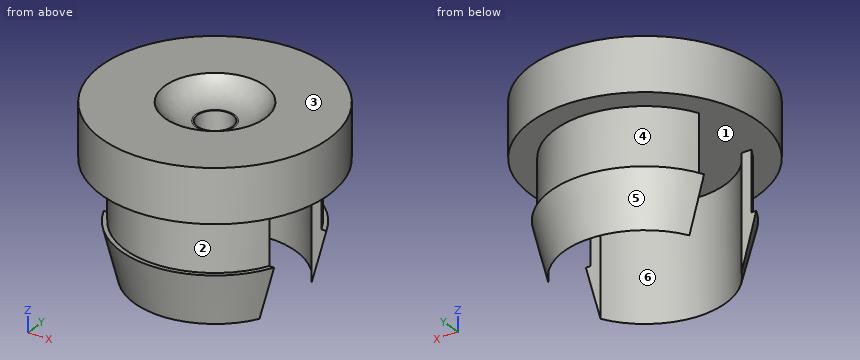
Autodesk Inventor part; units mm, degrees
ref_plane "XZ Plane" through (0, 0, 0) normal (0, 1, 0) x (-1, 0, 0)
ref_plane "XY Plane" through (0, 0, 0) normal (0, 0, 1) x (1, 0, 0)
sketch "Sketch1" plane through (0, 0, 0) normal (0, 0, 1) x (1, 0, 0)
  circle A0 centre (0, 0) radius 6.4
  dimension "d0" = 12.8
sketch "Sketch2" plane through (0, 0, 0) normal (0, 0, 1) x (1, 0, 0)
  circle A0 centre (0, 0) radius 2.825
  dimension "d3" = 5.65
sketch "Sketch3" plane through (0, 0, 0) normal (0, 0, 1) x (1, 0, 0)
  circle A0 centre (0, 0) radius 1
  dimension "d4" = 2
extrude "Extrusion1" add sketch "Sketch1" against normal blind 3
extrude "Extrusion2" cut sketch "Sketch2" against normal blind 1
extrude "Extrusion3" cut sketch "Sketch3" against normal blind 3
fillet "Fillet1" radius 2 1 edges at (-2.825, 0, -1)
sketch "Sketch4" plane through (0, 0, 0) normal (0, 1, 0) x (-1, 0, 0)
  line L0 (-5.0465, -3) -> (-5.0465, -6.35)
  line L1 (-6.4, -3) -> (6.4, -3)
  line L2 (-5.2965, -6.35) -> (-4.5465, -9.35)
  line L3 (-5.2965, -6.35) -> (-5.0465, -6.35)
  line L4 (-4.5465, -3) -> (-4.5465, -9.35)
  line L5 (-5.0465, -3) -> (-4.5465, -3)
  line L6 (0, -3) -> (0, -11.7949)
  point P0 (0, 0)
  dimension "d21" = 0.25
  dimension "d26" = 6.35
  dimension "d28" = 0.5
  dimension "d29" = 90
revolve "Revolution2" add sketch "Sketch4" angle 360 about axis through (0, 0, -3) along (0, 0, -1)
ref_plane "Work Plane2" through (6.4, 0, 0) normal (1, 0, 0) x (0, 1, 0)
sketch "Sketch7" plane through (6.4, 0, 0) normal (1, 0, 0) x (0, 1, 0)
  line L0 (-2.15, -3) -> (-2.15, -9.35)
  line L1 (-2.15, -9.35) -> (2.15, -9.35)
  line L2 (2.15, -9.35) -> (2.15, -3)
  line L3 (2.15, -3) -> (-2.15, -3)
  point P0 (0, 0)
  dimension "d34" = 4.3
  dimension "d35" = 6.35
extrude "Extrusion4" cut sketch "Sketch7" against normal blind 12.8
properties part number "Cable end barrel stop"
Here's how the part is built. I have some questions about the finished solid (model axes, mm). Face numbers are marked on the shaded views. A direction names the side the tool comes from. Coordinates: 2 decimals unless noted, no trailing zeros. Write each loop counter-clockwise with the first axis right and the second up, starting at its lowest first coordinate (ties: lowest second). Pieces come first, ordered by that corner, then holes. Notation, with made-up numbers: (50.25, 54) -> (67.25, 54) arc R14 cw to (67.25, 71) -> close; hole circle Ø9 at (89, 46.25). An arc over 180 degrees is marked (long way). Use a Markdown table: item, result. Add a question column.
(1) For the marked faces 4, 5 and 6, which set-ups out of +Z, -Z, +X, -X, +Y, -Y let a thin tool reach every point of the face, with its end or its side?
(2) If we section it at A-A, the plane z = -5.75: Write out the boundary of the cut face in (x, y), and give its area (3 significant figures).
(3) Please list where these lines run through material, in increasing order: line 1 (Y direction, x = 0, z = -2.05); line 2 (Z direction, x = 3, y = 0.5); line 3 (X direction, y = -2.25, z = -6.25).
(4) We'd pull the mould along Y, two halves only. Please class the marked faces 1, 2 and 3: +Y half, -Y half, draft (parallel to the pull), parting line (faces both ways), or undercut.
(5) I'm going to push flat-ended pins straight in: P1, Ø5, axis at y = -2.5, z = -6.5, coming from the +X side; P2, Ø4, axis at x = 0, z = -8.5, coming from the -Y side; P3, Ø1.7, axis at x = 0.5, y = -0.5, coming from the +Z side. Where does each tip first touch, or does it pass through?
(6) If we section it at B-B, the plane z = -1.25: Write out the boundary of the cut face in (x, y), and give its area (3 significant figures).
Outcome:
| question | item | result |
|---|---|---|
| 1 | face 4 | +Y |
| 1 | face 5 | -Z, +Y |
| 1 | face 6 | -Z |
| 2 | outline | (-4.57, -2.15) arc R5.05 ccw to (4.57, -2.15) -> (4.01, -2.15) arc R4.55 cw to (-4.01, -2.15) -> close; (-4.57, 2.15) -> (-4.01, 2.15) arc R4.55 cw to (4.01, 2.15) -> (4.57, 2.15) arc R5.05 ccw to start |
| 2 | area | 10.6 mm^2 |
| 3 | line 1 | y = -6.4 to -1, 1 to 6.4 |
| 3 | line 2 | z = -3 to 0 |
| 3 | line 3 | x = -4.52 to -3.95, 3.95 to 4.52 |
| 4 | face 1 | undercut |
| 4 | face 2 | -Y half |
| 4 | face 3 | draft |
| 5 | P1 | stops at x = 4.84 |
| 5 | P2 | stops at y = -5.26 |
| 5 | P3 | stops at z = -0.95 |
| 6 | outline | circle Ø12.8 at (0, 0); hole circle Ø2 at (0, 0) |
| 6 | area | 126 mm^2 |
